Design review of the part built by this model. Coordinates are the model's own, in mm. Face numbers are marked on the shaded views. A direction names the side the tool comes from. Give positions to 0.01 mm unless a question says otherwise; leave off trailing zeros. Loops run counter-clockwise (first coordinate to the right, second up) from the corner with the lowest first, then second, coordinate; pieces in that order, holes last. Notation, with made-up numbers: (0, -26.5) -> (37, -26.5) arc R32 cw to (37, 8.5) -> close; hole circle Ø1 at (44, -24.5). An arc over 180 degrees is marked (long way). Answer in a Markdown table with one row per item. Add a question column.
(1) Consider section C-C on y = 24.5. Write out the cut boundary in (x, z).
(2) Consider section B-B on x = -9. Write out the cut boundary in (y, z), then the cut area to 4 significant figures.
(3) Consider section D-D on y = -8. Write out the cut boundary in (x, z).
(4) For pin 1 (1.5 mm diameter, centred on x = 12, y = 29, fed in from +Z); pin 2 (1 mm diameter, centred on x = -7, y = 20, fed in from +Z); pin 3 (7.5 mm diameter, centred on x = -5.5, z = 9, fed in from +Y), all flat-tipped, find the tip position at first contact; note any pin that passes through.
(5) For the marked faces 1, 2 and 3, list the 3-axis set-ups (+Z, -Z, +X, -X, +Y, -Y) from which the entire face can be reached by the end or side of a thin tool; tool diameter is ignored.
(6) Consider section A-A on z = 10.5. Write out the cut boundary in (x, y).
(7) Draft analysis for pull direction Z (two halves, no side actions). For the marked faces 4 and 5, state which applies: +Z half, -Z half, draft (parallel to the pull), parting line (faces both ways), or undercut.
(8) For line 1 (X direction, y = 29, z = 14.75); line 2 (Y direction, x = -15.5, z = 11.75); line 3 (Y direction, x = 4, z = 6), list the stretches that pass through material, from the lowest coordinate up.
from build123d import *

# Parameters (mm, degrees)
F0_W     = 36
F0_H     = 74
F1_DEPTH = 4
F2_W     = 3
F2_H     = 13
F2_W_2   = 32
F2_H_2   = 3
F3_DEPTH = 12
F4_DEPTH = 15
F5_SIZE  = 1


with BuildPart() as f1:
    # F0 (on Top) → F1 (new body)
    with BuildSketch(Plane.XY):
        Rectangle(F0_W, F0_H)
    extrude(amount=F1_DEPTH)

    # F2 (on face) → F3 (join)
    with BuildSketch(Plane.XY.offset(4)):
        with Locations((-12.5, 27.5)):
            Rectangle(F2_W, F2_H)
        with Locations((12.5, 27.5)):
            Rectangle(F2_W, F2_H)
        with Locations((2, -31.5)):
            Rectangle(F2_W_2, F2_H_2)
    extrude(amount=F3_DEPTH)

    # F2 (on face) → F4 (join)
    with BuildSketch(Plane.XY.offset(4)):
        Polygon((-11, 37), (-18, 37), (-18, 21), (-14, 21), (-14, 34), (-11, 34), align=None)
        Polygon((18, 37), (11, 37), (11, 34), (14, 34), (14, 21), (18, 21), align=None)
        Polygon((-14, -30), (-18, -30), (-18, -37), (18, -37), (18, -33), (-14, -33), align=None)
    extrude(amount=F4_DEPTH)

    # F5
    f5_edges = [f1.edges().sort_by_distance(p)[0] for p in [
        (-14, 27.5, 19),
        (-12.5, 34, 19),
        (12.5, 34, 19),
        (14, 27.5, 19),
        (2, -33, 19),
        (-14, -31.5, 19),
    ]]
    chamfer(f5_edges, length=F5_SIZE)


solid = f1.part
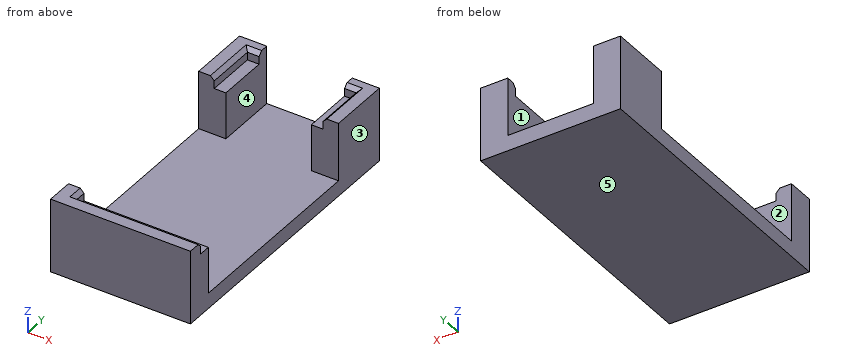
Values follow:
| question | item | result |
|---|---|---|
| 1 | outline | (-18, 0) -> (18, 0) -> (18, 19) -> (15, 19) -> (14, 18) -> (14, 16) -> (11, 16) -> (11, 4) -> (-11, 4) -> (-11, 16) -> (-14, 16) -> (-14, 18) -> (-15, 19) -> (-18, 19) -> close |
| 2 | outline | (-37, 0) -> (37, 0) -> (37, 4) -> (-30, 4) -> (-30, 16) -> (-33, 16) -> (-33, 18) -> (-34, 19) -> (-37, 19) -> close |
| 2 | area | 391.5 mm2 |
| 3 | outline | (-18, 0) -> (18, 0) -> (18, 4) -> (-18, 4) -> close |
| 4 | pin 1 | z = 16 |
| 4 | pin 2 | z = 4 |
| 4 | pin 3 | y = -30 |
| 5 | face 1 | +Z, +Y |
| 5 | face 2 | +Z, +X, -X |
| 5 | face 3 | +Z, -Z, +X, +Y, -Y |
| 6 | outline | (-18, -37) -> (18, -37) -> (18, -30) -> (-18, -30) -> close; (-18, 21) -> (-11, 21) -> (-11, 37) -> (-18, 37) -> close; (11, 21) -> (18, 21) -> (18, 37) -> (11, 37) -> close |
| 7 | face 4 | draft |
| 7 | face 5 | -Z half |
| 8 | line 1 | -18 to -11, 11 to 18 |
| 8 | line 2 | -37 to -30, 21 to 37 |
| 8 | line 3 | -37 to -30 |
